CAD build for the part. Positions are in the model's coordinates, mm. Round coordinates to 2 decimals unless told otherwise and drop trailing zeros. Loops run counter-clockwise (first coordinate to the right, second up) from the corner with the lowest first, then second, coordinate; pieces in that order, holes last. Notation, with made-up numbers: (5.25, -9.75) - (44.25, -9.75) arc R6 ccw to (44.25, 0.25) - close; hole circle Ø3 at (85.25, 6). An arc over 180 degrees is marked (long way). Use one line per item in the form item = value.
from build123d import *

# Parameters (mm, degrees)
SKETCH1_W           = 300
SKETCH1_H           = 50
SKETCH1_R           = 4
MAIN_DEPTH          = 10
SKETCH4_R           = 2.5
MOUNT_DEPTH         = 154.297097168
SKETCH2_R           = 11
SKETCH2_R_2         = 1.5
STEPPER_MOUNT_DEPTH = 154.297097168


with BuildPart() as part:
    # Sketch1 → main (new body)
    with BuildSketch(Plane(origin=(0, 0, 0), x_dir=(1, 0, 0), z_dir=(0, 1, 0))):
        with Locations((0, -5)):
            Rectangle(SKETCH1_W, SKETCH1_H)
        with Locations(Location((-100, 0, 0), (0, 0, 270))):
            Circle(SKETCH1_R, mode=Mode.SUBTRACT)
        with Locations(Location((100, 0, 0), (0, 0, 90))):
            Circle(SKETCH1_R, mode=Mode.SUBTRACT)
    extrude(amount=MAIN_DEPTH)

    # Sketch4 → mount (cut, through all)
    with BuildSketch(Plane(origin=(0, 10, 0), x_dir=(1, 0, 0), z_dir=(0, 1, 0))):
        with Locations(Location((-140, 5, 0), (0, 0, 270))):
            Circle(SKETCH4_R)
        with Locations(Location((-140, -15, 0), (0, 0, 90))):
            Circle(SKETCH4_R)
        with Locations(Location((140, -15, 0), (0, 0, 270))):
            Circle(SKETCH4_R)
        with Locations(Location((140, 5, 0), (0, 0, 90))):
            Circle(SKETCH4_R)
    extrude(amount=-MOUNT_DEPTH, mode=Mode.SUBTRACT)

    # Sketch2 → stepper_mount (cut, through all)
    with BuildSketch(Plane(origin=(0, 10, 0), x_dir=(1, 0, 0), z_dir=(0, 1, 0))):
        with Locations(Location((0, -1, 0), (0, 0, 270))):
            Circle(SKETCH2_R)
        with Locations(Location((15.5, -16.5, 0), (0, 0, 270))):
            Circle(SKETCH2_R_2)
        with Locations(Location((-15.5, -16.5, 0), (0, 0, 90))):
            Circle(SKETCH2_R_2)
        with Locations(Location((-15.5, 14.5, 0), (0, 0, 270))):
            Circle(SKETCH2_R_2)
        with Locations(Location((15.5, 14.5, 0), (0, 0, 90))):
            Circle(SKETCH2_R_2)
    extrude(amount=-STEPPER_MOUNT_DEPTH, mode=Mode.SUBTRACT)


solid = part.part
1) Two-plate mould, pull along Z, no slides. Class faces 1 (the flat face through (-2, 0, 16)), 2 (the cylindrical face through (137.52, 5.07, -4.67)), 3 (the flat face through (-2, 5, -20)): +Z half, -Z half, draft (parallel to the pull), parting line (faces both ways), or undercut.
Report:
face_1 = draft
face_2 = undercut
face_3 = -Z half
2) Flat gauge pins, fed straight in: pin 1 (6 mm diameter, centred on x = -140, z = 15, fed in from -Y); pin 2 (1.8 mm diameter, centred on x = -15.5, z = 16.5, fed in from +Y). Where does each tip first touch, or does it go through?
Report:
pin_1 = 0
pin_2 = through
3) Slice it at B-B (y = 7.25). State how many separate pieces and enclosed holes the cut face has, plus the area to 3 significant figures.
Report:
separate_pieces = 1
enclosed_holes = 11
area = 14,400 mm^2
4) Slice it at A-A (x = -100). Write the cut outline in (y, z), plus the area to 3 significant figures.
Report:
outline = (0, -20) - (10, -20) - (10, -4) - (0, -4) - close; (0, 4) - (10, 4) - (10, 30) - (0, 30) - close
area = 420 mm^2
5) Slice it at C-C (x = 140). Write the cut outline in (y, z).
Report:
outline = (0, -20) - (10, -20) - (10, -7.5) - (0, -7.5) - close; (0, -2.5) - (10, -2.5) - (10, 12.5) - (0, 12.5) - close; (0, 17.5) - (10, 17.5) - (10, 30) - (0, 30) - close
6) Drill centre lines: probe 1 along Z at (x, y) = (140, 3.5); probe 2 along X at (y, z) = (5, 14.5); probe 3 along X at (y, z) = (7, 0). Where is each one in solid material? Low to high.
Report:
probe_1 = -20 to -7.5, -2.5 to 12.5, 17.5 to 30
probe_2 = -150 to -142.45, -137.55 to 137.55, 142.45 to 150
probe_3 = -150 to -104, -96 to -10.95, 10.95 to 96, 104 to 150
